from build123d import *

# Parameters (mm, degrees)
F0_W      = 40
F0_H      = 35
F1_DEPTH  = 40
F2_SIZE   = 1
F5_D      = 16
F6_W      = 12
F6_H      = 8
F7_DEPTH  = 25
F8_W      = 10
F8_H      = 16
F9_DEPTH  = 13.7560020016
F11_D     = 6
F11_DEPTH = 20
F11_TIP   = 1.8025818571
F13_D     = 3.4
F13_DEPTH = 16
F13_TIP   = 1.0214630523
F15_D     = 5
F15_DEPTH = 21
F15_TIP   = 1.5021515476
F17_D     = 2.5
F17_DEPTH = 15.5
F17_TIP   = 0.7510757738


with BuildPart() as f1:
    # F0 (on Top) → F1 (new body)
    with BuildSketch(Plane.XY):
        Rectangle(F0_W, F0_H)
    extrude(amount=F1_DEPTH)

    # F2
    f2_edges = [f1.edges().sort_by_distance(p)[0] for p in [
        (0, -17.5, 40),
    ]]
    chamfer(f2_edges, length=F2_SIZE)

    # F5 (through all)
    with Locations(Plane.XY.offset(40)):
        with Locations((0, 2.5)):
            Hole(F5_D / 2)

    # F6 (on face) → F7 (cut)
    with BuildSketch(Plane.XZ.offset(17.5)):
        with Locations((0, 36)):
            Rectangle(F6_W, F6_H)
    extrude(amount=-F7_DEPTH, mode=Mode.SUBTRACT)

    # F8 (on face) → F9 (cut, through all)
    with BuildSketch(Plane.XZ.offset(17.5)):
        with Locations((0, 8)):
            Rectangle(F8_W, F8_H)
    extrude(amount=-F9_DEPTH, mode=Mode.SUBTRACT)

    # F11
    with Locations(Plane.XY.offset(40)):
        with Locations((13, 10.5), (-13, -10.5)):
            Hole(F11_D / 2, depth=F11_DEPTH)
            with Locations((0, 0, -(F11_DEPTH + F11_TIP / 2))):  # 118° drill point
                Cone(0, F11_D / 2, F11_TIP, mode=Mode.SUBTRACT)

    # F13
    with Locations(Plane(origin=(0, 0, 0), x_dir=(1, 0, 0), z_dir=(0, 0, -1))):
        with Locations((-13, -10.5), (13, 10.5)):
            Hole(F13_D / 2, depth=F13_DEPTH)
            with Locations((0, 0, -(F13_DEPTH + F13_TIP / 2))):  # 118° drill point
                Cone(0, F13_D / 2, F13_TIP, mode=Mode.SUBTRACT)

    # F15
    with Locations(Plane(origin=(0, 0, 0), x_dir=(1, 0, 0), z_dir=(0, 0, -1))):
        with Locations((-13, 10.5), (13, -10.5)):
            Hole(F15_D / 2, depth=F15_DEPTH)
            with Locations((0, 0, -(F15_DEPTH + F15_TIP / 2))):  # 118° drill point
                Cone(0, F15_D / 2, F15_TIP, mode=Mode.SUBTRACT)

    # F17
    with Locations(Plane.XY.offset(32)):
        with Locations((0, -11.5)):
            Hole(F17_D / 2, depth=F17_DEPTH)
            with Locations((0, 0, -(F17_DEPTH + F17_TIP / 2))):  # 118° drill point
                Cone(0, F17_D / 2, F17_TIP, mode=Mode.SUBTRACT)


solid = f1.part
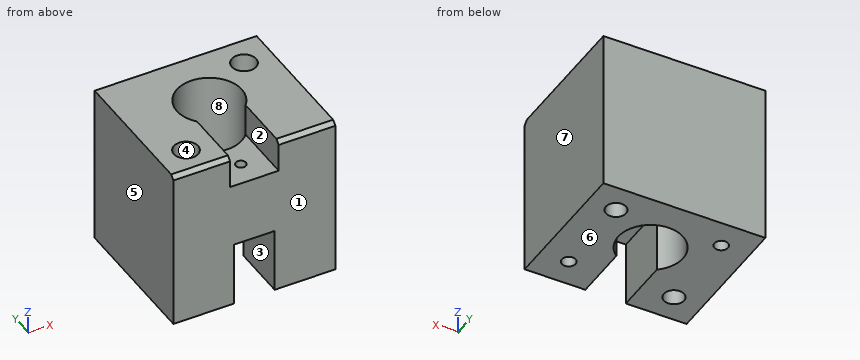
Model file for the job. Use its own axes, mm. Face numbers are marked on the shaded views. A direction names the side the tool comes from. Give positions to 0.01 mm unless a question says otherwise; leave off trailing zeros. Order: outer loops, then holes, each group sorted by start corner. A loop starts at its lowest first (then second) coordinate and runs counter-clockwise, first axis right, second up. Notation, with made-up numbers: (60.5, 9) - (118.5, 9) arc R29 ccw to (118.5, 47) - close; hole circle Ø5 at (39.5, -24.75). An arc over 180 degrees is marked (long way). One line per item, written item: value.
Item 1: Two-plate mould, pull along X, no slides. Class the marked faces 5, 6, 7 and 8: released by +X, released by -X, zero draft, split by the parting line, or undercut.
Response values:
face 5: released by -X
face 6: zero draft
face 7: released by +X
face 8: undercut
Item 2: Slice it at C-C (z = 33.5). List the corners of the cut face in (x, y), then the cut area to 3 significant figures.
Response values:
outline: (-20, -17.5) - (-6, -17.5) - (-6, -2.79) arc R8 cw (long way) to (6, -2.79) - (6, -17.5) - (20, -17.5) - (20, 17.5) - (-20, 17.5) - close; hole circle Ø6 at (-13, -10.5); hole circle Ø6 at (13, 10.5)
area: 988 mm2
Item 3: Slice it at A-A (z = 12.5). List the corners of the cut face in (x, y) (3 decimals), then the cut area to 3 significant figures.
Response values:
outline: (-20, -17.5) - (-5, -17.5) - (-5, -3.745) arc R8 cw (long way) to (5, -3.745) - (5, -17.5) - (20, -17.5) - (20, 17.5) - (-20, 17.5) - close; hole circle Ø5 at (-13, -10.5); hole circle Ø3.4 at (-13, 10.5); hole circle Ø5 at (13, 10.5); hole circle Ø3.4 at (13, -10.5)
area: 1,020 mm2
Item 4: Slice it at B-B (y = 2.5). List the corners of the cut face in (x, z).
Response values:
outline: (-20, 0) - (-8, 0) - (-8, 40) - (-20, 40) - close; (8, 0) - (20, 0) - (20, 40) - (8, 40) - close
Item 5: Slice it at D-D (y = 6). List the corners of the cut face in (x, z), then the cut area to 3 significant figures.
Response values:
outline: (-20, 0) - (-7.19, 0) - (-7.19, 40) - (-20, 40) - close; (7.19, 0) - (20, 0) - (20, 40) - (7.19, 40) - close
area: 1,020 mm2
Item 6: Tool access for the marked faces 1, 2, 3 and 4: list every direction of +Z, -Z, +X, -X, +Y, -Y with a clear straight run to the whole face (end or side of a thin tool).
Response values:
face 1: +Z, -Z, +X, -X, -Y
face 2: +Z, -Y
face 3: -Z, -Y
face 4: +Z
Item 7: Wall check: line 1 (Y direction, x = 0, z = 25.5); line 2 (Y direction, x = 13, z = 11.5); line 3 (X direction, y = -10.5, z = 12.5). Give the ranges that are in metal, low to high.
Response values:
line 1: -17.5 to -12.75, -10.25 to -5.5, 10.5 to 17.5
line 2: -17.5 to -12.2, -8.8 to 8, 13 to 17.5
line 3: -20 to -15.5, -10.5 to -5, 5 to 11.3, 14.7 to 20
Item 8: Pin check, flat tips, straight feed: pin 1 Ø5 at (x, y) = (-4.5, 0) entering from +Z; pin 2 Ø2 at (x, y) = (0, -11.5) entering from -Z; pin 3 Ø3.5 at (x, y) = (0.5, -11) entering from +Z. Stop position of each tip, or through.
Response values:
pin 1: through
pin 2: z = 16
pin 3: z = 32
